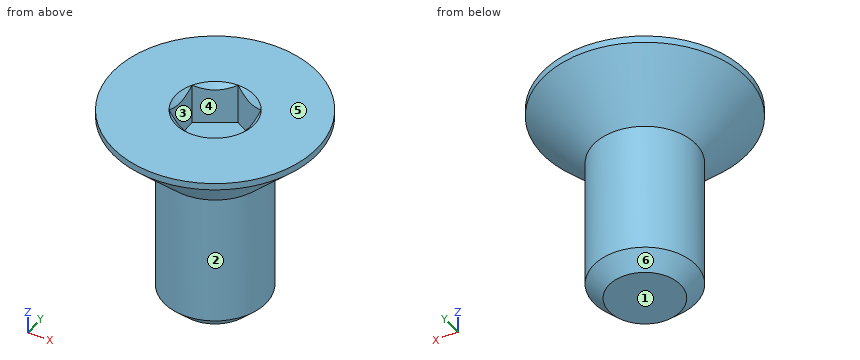
```python
from build123d import *

# Parameters (mm, degrees)
SKETCH3_W          = 6
SKETCH3_H          = 1.5
CHAMFER1_SIZE      = 0.45
CUT_EXTRUDE1_DEPTH = 1.19


with BuildPart() as part:
    # Sketch3 → Revolve1 (revolve)
    with BuildSketch(Plane(origin=(0, 0, 0), x_dir=(0, 0, -1), z_dir=(1, 0, 0))):
        with Locations((0, 0.75)):
            Rectangle(SKETCH3_W, SKETCH3_H)
    revolve(axis=Axis((0, 0, -3), (0, 0, 1)))

    # Chamfer1
    chamfer1_edges = [part.edges().sort_by_distance(p)[0] for p in [
        (0, -1.5, -3),
    ]]
    chamfer(chamfer1_edges, length=CHAMFER1_SIZE)

    # Sketch6 → Revolve2 (revolve)
    with BuildSketch(Plane(origin=(0, 0, 0), x_dir=(0, 0, -1), z_dir=(1, 0, 0))):
        Polygon((-3, 3), (-2.8, 3), (-1.3, 1.5), (-1.3, 0), (-3, 0), align=None)
    revolve(axis=Axis((0, 0, -3), (0, 0, 1)))

    # Sketch8 → Cut-Extrude1 (cut)
    with BuildSketch(Plane.XY.offset(3)):
        Polygon((0, 1.154700538), (-1, 0.577350269), (-1, -0.577350269), (0, -1.154700538), (1, -0.577350269), (1, 0.577350269), align=None)
    extrude(amount=-CUT_EXTRUDE1_DEPTH, mode=Mode.SUBTRACT)

    # Cut-Extrude2 cone 1 section (through the dimple's axis) → Cut-Extrude2 (revolve, cut)
    with BuildSketch(Plane(origin=(0, 0, 3), x_dir=(0, -1, 0), z_dir=(1, 0, 0))):
        Polygon((0, 0), (1.154700538, 0), (0, 1.154700538), align=None)
    revolve(axis=Axis((0, 0, 3), (0, 0, -1)), mode=Mode.SUBTRACT)


solid = part.part
```
Can you work these out from the model? Positions are in its coordinate system, mm. Face numbers are marked on the shaded views. A direction names the side the tool comes from. Round coordinates to 2 decimals unless told otherwise and drop trailing zeros. Loops run counter-clockwise (first coordinate to the right, second up) from the corner with the lowest first, then second, coordinate; pieces in that order, holes last. Notation, with made-up numbers: M 49.5,43 L 79.5,43 A18 ccw 79.5,54 Z; hole C 18.5,-21 d4. An arc over 180 degrees is marked long. Write item = value, one per line. Start each with the question number.
(1) Suppose I cut it at C-C on z = 0. Write out the boundary of the cut face in (x, y).
(2) Suppose I cut it at B-B on y = 0. Write out the boundary of the cut face in (x, z), plus the area to 3 significant figures.
(3) Which directions (+Z, -Z, +X, -X, +Y, -Y) give clear straight access to the entire face, cutting with the end or side of a thin tool? Please do the marked faces 1, 2 and 3.
(4) If we mould it in two halves opening along X, with no side actions, what happens to the marked faces 4, 5 and 6? For each: released by +X, released by -X, zero draft, split by the parting line, or undercut.
(5) I'm going to push flat-ended pins straight in: P1, Ø3, axis at x = -2, z = 2, coming from the -Y side; P2, Ø3, axis at y = 1, z = 1, coming from the -X side; P3, Ø3, axis at y = -1.5, z = -1, coming from the +X side. Where does each tip first touch, or does it pass through?
(6) Suppose I cut it at A-A on z = 2.2. Write out the boundary of the cut face in (x, y).
(7) I need wall thicknesses on line 1 along X through (y, z) = (0.55, 2.1); line 2 along X through (y, z) = (0.6, -2.05); line 3 along X through (y, z) = (-0.1, 0.5). Which ranges of each line are inside material? Lowest first, please.
Answer block:
q1.outline = C 0,0 d3
q2.outline = M -3,2.8 L -1.5,1.3 L -1.5,-2.55 L -1.05,-3 L 1.05,-3 L 1.5,-2.55 L 1.5,1.3 L 3,2.8 L 3,3 L 1.15,3 L 1,2.85 L 1,1.81 L -1,1.81 L -1,2.85 L -1.15,3 L -3,3 Z
q2.area = 18.2 mm²
q3.face_1 = -Z, +X, -X, +Y, -Y
q3.face_2 = -Z
q3.face_3 = +Z
q4.face_4 = undercut
q4.face_5 = zero draft
q4.face_6 = split by the parting line
q5.P1 = -2.91
q5.P2 = -2.58
q5.P3 = 1.5
q6.outline = C 0,0 d4.8; hole M -1,-0.58 L 0,-1.15 L 1,-0.58 L 1,0.58 L 0,1.15 L -1,0.58 Z
q7.line_1 = -2.23 to -1, 1 to 2.23
q7.line_2 = -1.37 to 1.37
q7.line_3 = -1.5 to 1.5
